Source: CAD feature listing. Evaluate the final solid. Frame: model axes, mm. A direction names the side the tool comes from. Coordinates: 2 decimals unless noted, no trailing zeros. Write each loop counter-clockwise with the first axis right and the second up, starting at its lowest first coordinate (ties: lowest second). Pieces come first, ordered by that corner, then holes. Notation, with made-up numbers: M -16,38 L -11,38 A32 ccw -11,73 Z; hole C 25,39 d8. An arc over 180 degrees is marked long. Write item = value, one per line. Start each with the question number.
1. Pull-direction query (X, two-part tool) for faces 1 (the face through (-18, 0, 980)), 2 (the face through (20, 0, 493)), 3 (the face through (-20, 0, 493)), 4 (the face through (0, -17, 493)); classes: pulls with the +X half, pulls with the -X half, needs draft (parallel to the pull), parting line crosses it, or undercut.
2. Section query A-A (y = 9). Output: boundary loops of the cut face in (x, z).
3. Access query for faces 5 (the face through (0, 17, 493)), 6 (the face through (-18, 0, 20)). Directions: +Z, -Z, +X, -X, +Y, -Y. A direction counts if a zero-diameter tool reaches every point of the face in a straight line with its end or side. Return the directions, or none.
4. Line query: line 1 along X through (y, z) = (-2, 145); line 2 along Y through (x, z) = (18, 389.5). Output: solid intervals per line, ascending.
5. Section query C-C (z = 310.5). Output: boundary loops of the cut face in (x, y), then the cut area to 3 significant figures.
Autodesk Inventor part; units mm, degrees
ref_plane "Start Plane" through (0, 0, 20) normal (0, 0, 1) x (1, 0, 0)
ref_plane "End Plane" through (0, 0, 980) normal (0, 0, 1) x (1, 0, 0)
ref_plane "Work Plane4" through (-15.5, 1520, 20) normal (0, 0, -1) x (-1, 0, 0)
ref_plane "Start Plane" through (0, 0, 20) normal (0, 0, 1) x (1, 0, 0)
ref_plane "End Plane" through (0, 0, 980) normal (0, 0, 1) x (1, 0, 0)
sketch "Sketch" plane through (0, 0, 0) normal (0, 0, 1) x (1, 0, 0)
  line L0 (-20, -15.5) -> (-20, 15.5)
  line L1 (-15.5, 20) -> (15.5, 20)
  line L2 (20, 15.5) -> (20, -15.5)
  line L3 (15.5, -20) -> (-15.5, -20)
  arc A0 (-20, -15.5) -> (-15.5, -20) centre (-15.5, -15.5) ccw
  arc A1 (-15.5, 20) -> (-20, 15.5) centre (-15.5, 15.5) ccw
  arc A2 (20, 15.5) -> (15.5, 20) centre (15.5, 15.5) ccw
  arc A3 (15.5, -20) -> (20, -15.5) centre (15.5, -15.5) ccw
  arc A4 (-15.5, 17) -> (-17, 15.5) centre (-15.5, 15.5) ccw
  line L4 (-15.5, 17) -> (15.5, 17)
  arc A5 (17, 15.5) -> (15.5, 17) centre (15.5, 15.5) ccw
  line L5 (17, 15.5) -> (17, -15.5)
  arc A6 (15.5, -17) -> (17, -15.5) centre (15.5, -15.5) ccw
  line L6 (15.5, -17) -> (-15.5, -17)
  arc A7 (-17, -15.5) -> (-15.5, -17) centre (-15.5, -15.5) ccw
  line L7 (-17, -15.5) -> (-17, 15.5)
  line L8 (0, 29.3048) -> (0, -29.3048) construction
  line L9 (-29.3048, 0) -> (29.3048, 0) construction
  dimension "d7" = 4.5
  dimension "d10" = 40
  dimension "d11" = 40
  dimension "d12" = 3
  dimension "d15" = 20
  dimension "d16" = 20
extrude "Body" add sketch "Sketch" along normal up to surface (960 mm away) from surface at 20
sketch "Sketch3" plane through (0, 0, 0) normal (0, 0, 1) x (1, 0, 0)
  line L0 (0, 0) -> (10, 0)
ref_plane "Work Plane3" through (0, 0, 0) normal (0, -1, 0) x (1, 0, 0)
ref_plane "Work Plane4" through (-15.5, 1520, 20) normal (0, 0, -1) x (-1, 0, 0)
split "Split1" plane through (-15.5, 1520, 20) removes the side toward (0, 0, -1)
ref_plane "Work Plane5" through (15.5, 1520, 980) normal (0, 0, 1) x (1, 0, 0)
split "Split2" plane through (15.5, 1520, 980) removes the side toward (0, 0, 1)
sketch "Sketch4" plane through (0, 0, 0) normal (0, -1, 0) x (1, 0, 0)
  line L0 (-2, 20) -> (12, 20)
  line L1 (-2, 980) -> (12, 980)
  dimension "d18" = 960
equation "\"d7\" = G_IR"
equation "\"d10\" = G_H"
equation "\"d11\" = G_W"
equation "\"d12\" = G_T"
equation "\"d15\" = 0.5 * d10"
equation "\"d16\" = 0.5 * d11"
equation "\"d3\" = G_L"
equation "\"G_W\" = 40"
equation "\"G_H\" = 40"
equation "\"G_T\" = 3"
equation "\"G_IR\" = 4.5"
equation "\"G_L\" = d18"
properties part number "ISO 12633-2 - 40x40x3 - 960" material "Steel, Mild"
Results are:
q1.face_1 = needs draft
q1.face_2 = pulls with the +X half
q1.face_3 = pulls with the -X half
q1.face_4 = undercut
q2.outline = M -20,20 L -17,20 L -17,980 L -20,980 Z; M 17,20 L 20,20 L 20,980 L 17,980 Z
q3.face_5 = +Z, -Z
q3.face_6 = -Z, +X, -X, +Y, -Y
q4.line_1 = -20 to -17, 17 to 20
q4.line_2 = -19.24 to 19.24
q5.outline = M -20,-15.5 A4.5 ccw -15.5,-20 L 15.5,-20 A4.5 ccw 20,-15.5 L 20,15.5 A4.5 ccw 15.5,20 L -15.5,20 A4.5 ccw -20,15.5 Z; hole M -17,-15.5 A1.5 ccw -15.5,-17 L 15.5,-17 A1.5 ccw 17,-15.5 L 17,15.5 A1.5 ccw 15.5,17 L -15.5,17 A1.5 ccw -17,15.5 Z
q5.area = 429 mm^2
